Read the model definition and answer for the solid it produces. Units are mm, in the model's axes. Face numbers are marked on the shaded views. A direction names the side the tool comes from. Give positions to 0.01 mm unless a question says otherwise; leave off trailing zeros. Loops run counter-clockwise (first coordinate to the right, second up) from the corner with the lowest first, then second, coordinate; pieces in that order, holes last. Notation, with made-up numbers: (76.25, 66.25) - (98.25, 66.25) arc R24 cw to (98.25, 79.25) - close; hole circle Ø1 at (9.25, -34). An arc over 180 degrees is marked (long way). Write each question's results on one line, items separated by ' | '. Start each with the question number.
Q1. Given pin 1 (3 mm diameter, centred on x = -22, y = 7.5, fed in from -Z); pin 2 (4.5 mm diameter, centred on y = 9, z = 32.5, fed in from -X); pin 3 (2 mm diameter, centred on x = -17, y = 16.5, fed in from +Z), each flat-ended and moving along its own axis, determine where each tip first touches the part or whether it passes through.
Q2. The part is cut by section A-A, the plane y = 15.5. Write down the section's boundary in (x, z), plus the area to 3 significant figures.
Q3. Find the intervals of material crossed by line 1 (Z direction, x = -27.5, y = 19); line 2 (Z direction, x = -6, y = 14.5); line 3 (X direction, y = 17.75, z = -0.5), in increasing order. Write a range as from..to.
Q4. The part is cut by section B-B, the plane y = 12.75. Write down the section's boundary in (x, z).
Q5. The part is cut by section C-C, the plane z = 1. Write down the section's boundary in (x, y).
Q6. The part is cut by section D-D, the plane x = -9. Write down the section's boundary in (y, z), plus the area to 3 significant figures.
Q7. For the marked faces 1 and 2, determine the directions among +Z, -Z, +X, -X, +Y, -Y from which every point of the face is accessible in a straight line to the end or side of a thin tool.
```python
from build123d import *

# Parameters (mm, degrees)
EXTRUDE_2_DEPTH     = 20
SKETCH_2_W          = 2
SKETCH_2_H          = 10
EXTRUDE_3_DEPTH     = 20
FILLET_1_R          = 2
SKETCH_3_R          = 2.1
CUT_EXTRUDE_1_DEPTH = 20
FILLET_2_R          = 2


with BuildPart() as part:
    # 草图1 → 凸台-拉伸2 (new body)
    with BuildSketch(Plane(origin=(0, 0, 0), x_dir=(1, 0, 0), z_dir=(0, 1, 0))):
        with BuildLine():
            ThreePointArc((0, -20.77807044), (-4.862027432, -9.040097872), (-16.6, -4.17807044))
            Line((-16.6, -4.17807044), (-30.2, -4.17807044))
            Line((-30.2, -4.17807044), (-30.2, -7.17807044))
            Line((-30.2, -7.17807044), (-26.118403227, -7.17807044))
            ThreePointArc((-26.118403227, -7.17807044), (-27.268887689, -8.060569291), (-28.337972568, -9.040097872))
            Line((-28.337972568, -9.040097872), (-26.216652224, -11.161418216))
            ThreePointArc((-26.216652224, -11.161418216), (-25.340775456, -10.358912872), (-24.398209873, -9.635901765))
            ThreePointArc((-24.398209873, -9.635901765), (-20.688184562, -7.807074064), (-16.6, -7.17807044))
            ThreePointArc((-16.6, -7.17807044), (-6.983347776, -11.161418216), (-3, -20.77807044))
            ThreePointArc((-3, -20.77807044), (-3.629003624, -24.866255002), (-5.457831325, -28.576280313))
            ThreePointArc((-5.457831325, -28.576280313), (-6.180842432, -29.518845896), (-6.983347776, -30.394722664))
            Line((-6.983347776, -30.394722664), (-4.862027432, -32.516043007))
            ThreePointArc((-4.862027432, -32.516043007), (-3.882498851, -31.446958129), (-3, -30.296473667))
            Line((-3, -30.296473667), (-3, -34.37807044))
            Line((-3, -34.37807044), (0, -34.37807044))
            Line((0, -34.37807044), (0, -20.77807044))
        make_face()
    extrude(amount=EXTRUDE_2_DEPTH)

    # 草图2 → 凸台-拉伸3 (add)
    with BuildSketch(Plane(origin=(0, 20, 0), x_dir=(1, 0, 0), z_dir=(0, 1, 0))):
        with Locations((-29.2, 0.82192956)):
            Rectangle(SKETCH_2_W, SKETCH_2_H)
    extrude(amount=-EXTRUDE_3_DEPTH)

    # 圆角1
    fillet_1_edges = [part.edges().sort_by_distance(p)[0] for p in [
        (-28.2, 10, 4.17807044),
    ]]
    fillet(fillet_1_edges, radius=FILLET_1_R)

    # 草图3 → 切除-拉伸1 (cut)
    with BuildSketch(Plane(origin=(-28.2, 0, 0), x_dir=(0, 0, -1), z_dir=(1, 0, 0))):
        with Locations((1.82192956, 15.5)):
            Circle(SKETCH_3_R)
        with Locations((1.82192956, 4.5)):
            Circle(SKETCH_3_R)
    extrude(amount=-CUT_EXTRUDE_1_DEPTH, mode=Mode.SUBTRACT)

    # 圆角2
    fillet_2_edges = [part.edges().sort_by_distance(p)[0] for p in [
        (-30.2, 10, 7.17807044),
    ]]
    fillet(fillet_2_edges, radius=FILLET_2_R)


solid = part.part
```
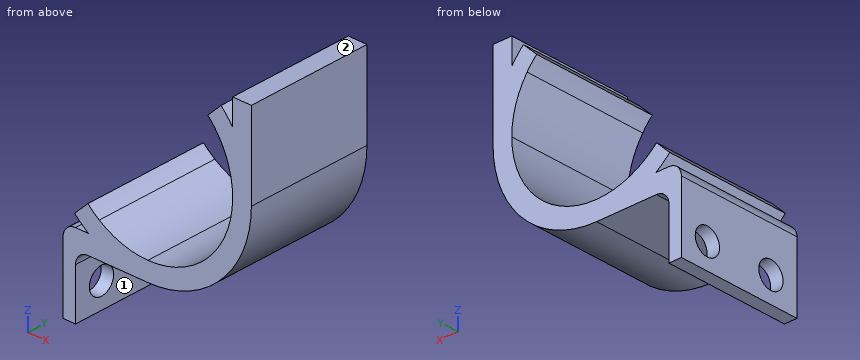
Check sheet entries:
1) pin 1: stops at z = 4.18 | pin 2: stops at x = -6.98 | pin 3: stops at z = 7.25
2) outline: (-30.2, -5.82) - (-28.2, -5.82) - (-28.2, -3.92) - (-30.2, -3.92) - close; (-30.2, 0.28) - (-28.2, 0.28) - (-28.2, 2.18) arc R2 cw to (-26.2, 4.18) - (-16.6, 4.18) arc R16.6 ccw to (0, 20.78) - (0, 34.38) - (-3, 34.38) - (-3, 30.3) arc R16.6 ccw to (-4.86, 32.52) - (-6.98, 30.39) arc R13.6 cw to (-26.22, 11.16) - (-28.34, 9.04) arc R16.6 ccw to (-26.12, 7.18) - (-28.2, 7.18) arc R2 ccw to (-30.2, 5.18) - close | area: 197 mm^2
3) line 1: z = 3.7..7.18, 8.26..9.88 | line 2: z = 8..12.26, 29.3..31.38 | line 3: x = -30.2..-28.2
4) outline: (-30.2, -5.82) - (-28.2, -5.82) - (-28.2, 2.18) arc R2 cw to (-26.2, 4.18) - (-16.6, 4.18) arc R16.6 ccw to (0, 20.78) - (0, 34.38) - (-3, 34.38) - (-3, 30.3) arc R16.6 ccw to (-4.86, 32.52) - (-6.98, 30.39) arc R13.6 cw to (-26.22, 11.16) - (-28.34, 9.04) arc R16.6 ccw to (-26.12, 7.18) - (-28.2, 7.18) arc R2 ccw to (-30.2, 5.18) - close
5) outline: (-30.2, 0) - (-28.2, 0) - (-28.2, 20) - (-30.2, 20) - close
6) outline: (0, 6.02) - (20, 6.02) - (20, 9.5) - (0, 9.5) - close | area: 69.6 mm^2
7) face 1: -Z, +X, +Y, -Y | face 2: +Z, +X, -X, +Y, -Y
